from build123d import *

# Parameters (mm, degrees)
BOX325_W     = 12
BOX325_H     = 10
BOX325_DEPTH = 13
BOX297_W     = 30
BOX297_H     = 65
BOX297_DEPTH = 13


with BuildPart() as box325:
    # Box325 → Box325 (new body)
    with BuildSketch(Plane(origin=(-85, -32, 34), x_dir=(1, 0, 0), z_dir=(0, 0, 1))):
        with Locations((6, 5)):
            Rectangle(BOX325_W, BOX325_H)
    extrude(amount=BOX325_DEPTH)


with BuildPart() as coral:
    # Box297 → Box297 (new body)
    with BuildSketch(Plane(origin=(-94, -22, 34), x_dir=(1, 0, 0), z_dir=(0, 0, 1))):
        with Locations((15, 32.5)):
            Rectangle(BOX297_W, BOX297_H)
    extrude(amount=BOX297_DEPTH)

    # Fusion197: union Box325
    add(box325.part)


solid = coral.part
The listing builds one solid part. Answer for the finished solid, in the listing's coordinates (mm). A direction names the side the tool comes from. Coordinates: 2 decimals unless noted, no trailing zeros. Order: outer loops, then holes, each group sorted by start corner. A loop starts at its lowest first (then second) coordinate and runs counter-clockwise, first axis right, second up.
Q1. Consider line 1 (Y direction, x = -90.5, z = 38.25); line 2 (X direction, y = -26, z = 45). Determine where each line is inside the solid, lowest interval first.
Q2. Which of the six approach directions +Z, -Z, +X, -X, +Y, -Y give full straight-line access (tool end or side, diameter ignored) to faces 1 (the face through (-90, -22, 40)), 2 (the face through (-79, 43, 40)), 3 (the face through (-73, -27, 40))?
Q3. Given P1, Ø2.5, axis at x = -68, z = 38, coming from the -Y side, flat-ended and moving along its own axis, determine where the tip first touches the part or whether it passes through.
Q4. A cutting plane is placed at B-B, the plane x = -91.5. Write down the section's boundary in (y, z).
Q5. A cutting plane is placed at A-A, the plane z = 36.5. Write down the section's boundary in (x, y), and give its area (3 significant figures).
Answers follow:
1. line 1: y = -22 to 43
1. line 2: x = -85 to -73
2. face 1: +Z, -Z, -X, -Y
2. face 2: +Z, -Z, +X, -X, +Y
2. face 3: +Z, -Z, +X, -Y
3. P1: stops at y = -22
4. outline: (-22, 34) - (43, 34) - (43, 47) - (-22, 47) - close
5. outline: (-94, -22) - (-85, -22) - (-85, -32) - (-73, -32) - (-73, -22) - (-64, -22) - (-64, 43) - (-94, 43) - close
5. area: 2,070 mm2
